Geometry check sheet. Reference: drawing and pictorial views, mm from the part's lowest x, y, z. A direction names the side the tool comes from. Coordinates: 2 decimals unless noted, no trailing zeros. Loops run counter-clockwise (first coordinate to the right, second up) from the corner with the lowest first, then second, coordinate; pieces in that order, holes last. Notation, with made-up numbers: (39.5, -36.5) - (83.5, -36.5) arc R19 cw to (83.5, -15.5) - close; hole circle Ø2 at (34.5, 30). An arc over 180 degrees is marked (long way). Use a Markdown table: item, result. Add a question column.
1) Sectioned sample at A-A, the plane y = 69.85. Enter the section's corners in (x, z) (3 decimals).
2) Draft check along Y on the marked faces 4, 5 and 6. Enter one of: pulls with the +Y half, pulls with the -Y half, needs draft (parallel to the pull), parting line crosses it, or undercut.
3) Sectioned sample at B-B, the plane z = 59.5. Enter the section's corners in (x, y).
4) Thickness scan on line 1 (Z direction, x = 40, y = 69.85) (3 decimals); line 2 (Y direction, x = 15, z = 69.85); line 3 (X direction, y = 93, z = 95.5). Record the ranges inside material, lowest first.
5) Go/stop test with flat-tipped pins: P1, Ø12, axis at y = 55.5, z = 55, coming from the +X side; P2, Ø2, axis at x = 61, z = 48.5, coming from the -Y side; P3, Ø3, axis at x = 46.5, z = 84.5, coming from the +Y side. Record where each tip stops, or that it passes through.
6) Sectioned sample at C-C, the plane x = 37. Enter the section's corners in (y, z) (3 decimals), then the cut area to 3 significant figures.
7) Sectioned sample at D-D, the plane x = 85.5. Enter the section's corners in (y, z), then the cut area to 3 significant figures.
8) Tool access check on the marked faces 1, 2 and 3. Record the directions out of +Z, -Z, +X, -X, +Y, -Y that give a thin tool (end or side, any length) a straight path to the whole face; none if there is none.
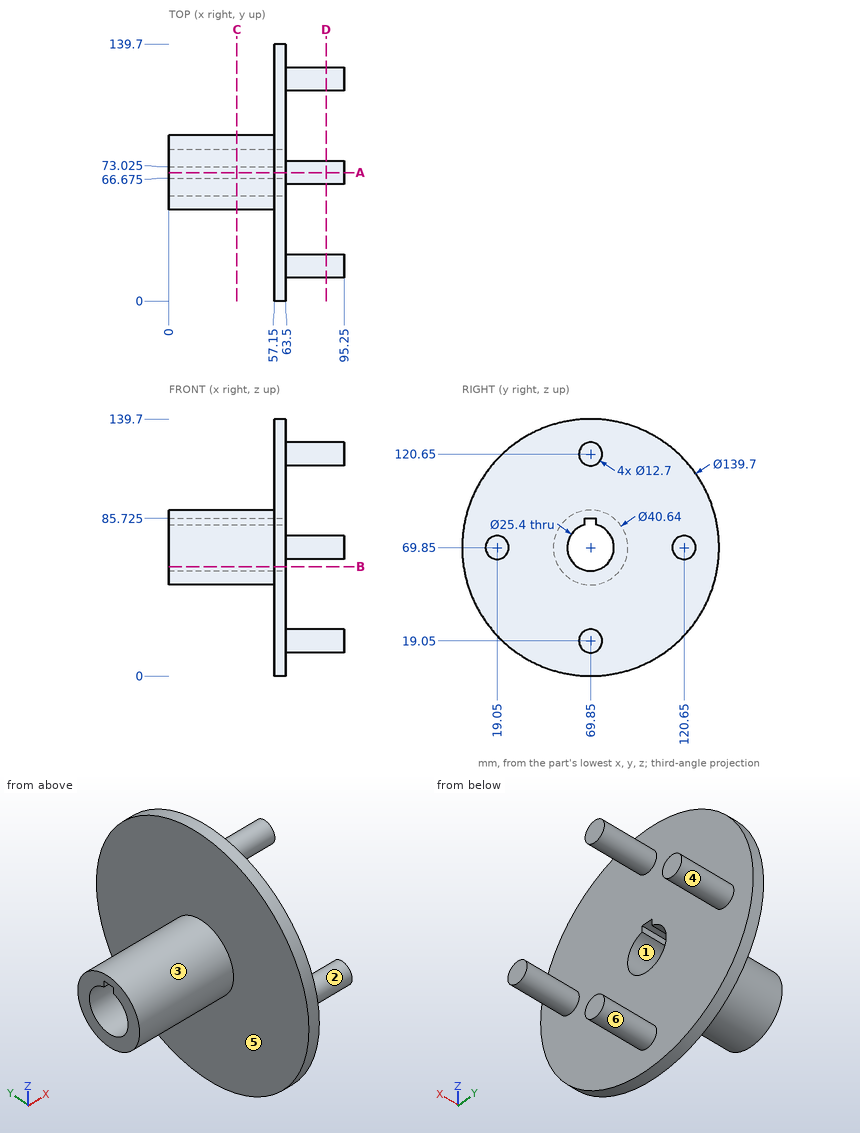
Solved:
| question | item | result |
|---|---|---|
| 1 | outline | (0, 49.53) - (57.15, 49.53) - (57.15, 0) - (63.5, 0) - (63.5, 12.7) - (95.25, 12.7) - (95.25, 25.4) - (63.5, 25.4) - (63.5, 57.15) - (0, 57.15) - close; (0, 85.725) - (63.5, 85.725) - (63.5, 114.3) - (95.25, 114.3) - (95.25, 127) - (63.5, 127) - (63.5, 139.7) - (57.15, 139.7) - (57.15, 90.17) - (0, 90.17) - close |
| 2 | face 4 | undercut |
| 2 | face 5 | needs draft |
| 2 | face 6 | parting line crosses it |
| 3 | outline | (0, 52.36) - (57.15, 52.36) - (57.15, 0.77) - (63.5, 0.77) - (63.5, 62.49) - (0, 62.49) - close; (0, 77.21) - (63.5, 77.21) - (63.5, 138.93) - (57.15, 138.93) - (57.15, 87.34) - (0, 87.34) - close |
| 4 | line 1 | z = 49.53 to 57.15, 85.725 to 90.17 |
| 4 | line 2 | y = 49.53 to 57.15, 82.55 to 90.17 |
| 4 | line 3 | x = 57.15 to 63.5 |
| 5 | P1 | stops at x = 63.5 |
| 5 | P2 | stops at y = 3.03 |
| 5 | P3 | stops at y = 85.34 |
| 6 | outline | circle Ø40.64 at (69.85, 69.85); hole (66.675, 82.147) arc R12.7 ccw (long way) to (73.025, 82.147) - (73.025, 85.725) - (66.675, 85.725) - close |
| 6 | area | 769 mm2 |
| 7 | outline | circle Ø12.7 at (19.05, 69.85); circle Ø12.7 at (69.85, 19.05); circle Ø12.7 at (69.85, 120.65); circle Ø12.7 at (120.65, 69.85) |
| 7 | area | 507 mm2 |
| 8 | face 1 | +X, -X |
| 8 | face 2 | +X |
| 8 | face 3 | -X |
